Design review of the part built by this model. Coordinates are the model's own, in mm. A direction names the side the tool comes from. Give positions to 0.01 mm unless a question says otherwise; leave off trailing zeros. Write each loop counter-clockwise with the first axis right and the second up, starting at its lowest first coordinate (ties: lowest second). Pieces come first, ordered by that corner, then holes. Notation, with made-up numbers: (-33, -10.5) -> (-2, -10.5) arc R28 ccw to (-2, 21.5) -> close; hole circle Ø5 at (44, 3). An arc over 180 degrees is marked (long way). Answer as a JSON object with one key per item and string values.
```python
from build123d import *

# Parameters (mm, degrees)
SKETCH_1_W               = 150
SKETCH_1_H               = 60
EXTRUDE_1_DEPTH          = 30
CUT_EXTRUDE_1_DEPTH      = 100
CUT_EXTRUDE_2_DEPTH      = 165.316767252
CUT_EXTRUDE_2_DEPTH_BACK = 165.316767252
SKETCH_5_R               = 2.05


with BuildPart() as part:
    # 스케치1 → 보스-돌출1 (new, symmetric)
    with BuildSketch(Plane(origin=(0, 0, 0), x_dir=(0, 0, -1), z_dir=(1, 0, 0))):
        with Locations((75, -30)):
            Rectangle(SKETCH_1_W, SKETCH_1_H)
    extrude(amount=EXTRUDE_1_DEPTH, both=True)

    # 스케치4 → 컷-돌출1 (cut)
    with BuildSketch(Plane.XY):
        with BuildLine():
            Line((-22.575, -30), (-22.575, -60))
            Line((-22.575, -60), (22.575, -60))
            Line((22.575, -60), (22.575, -30))
            ThreePointArc((22.575, -30), (0, -7.425), (-22.575, -30))
        make_face()
    extrude(amount=-CUT_EXTRUDE_1_DEPTH, mode=Mode.SUBTRACT)

    # 스케치5 → 컷-돌출2 (cut, two sides: drawn at the far end of the back side and taken through both)
    with BuildSketch(Plane(origin=(0, 0, 0), x_dir=(0, 0, -1), z_dir=(1, 0, 0)).offset(-CUT_EXTRUDE_2_DEPTH_BACK)):
        with Locations((107.446436282, -43.174787846)):
            Circle(SKETCH_5_R)
        with Locations((139.331395941, -33.939123257)):
            Circle(SKETCH_5_R)
    extrude(amount=CUT_EXTRUDE_2_DEPTH + CUT_EXTRUDE_2_DEPTH_BACK, mode=Mode.SUBTRACT)


solid = part.part
```
(1) We need section A-A, the plane x = 0. State the section outline as (y, z) points (3 decimals), then the cut area to 3 significant figures.
Here are the results:
{"outline": "(-60, -150) -> (0, -150) -> (0, 0) -> (-7.425, 0) -> (-7.425, -100) -> (-60, -100) -> close; hole circle Ø4.1 at (-43.175, -107.446); hole circle Ø4.1 at (-33.939, -139.331)", "area": "3,720 mm²"}
(2) We need section C-C, the plane y = -55. State the section outline as (x, z) points (3 decimals), then the cut area to 4 significant figures.
Here are the results:
{"outline": "(-30, -150) -> (30, -150) -> (30, 0) -> (22.575, 0) -> (22.575, -100) -> (-22.575, -100) -> (-22.575, 0) -> (-30, 0) -> close", "area": "4,485 mm²"}
(3) For line 1 along Z through (x, y) = (-18, -43.5); line 2 along X through (y, z) = (-54.5, -67) (3 decimals); line 3 along Z through (x, y) = (-18, -34), list the stretches that pass through material, from the lowest coordinate up.
Here are the results:
{"line 1": "z = -150 to -109.47, -105.42 to -100", "line 2": "x = -30 to -22.575, 22.575 to 30", "line 3": "z = -150 to -141.38, -137.28 to -100"}
(4) The part is to be moulded in two halves that separate along Y. For faces 3 (the flat face through (30, -30, -74)), 4 (the cylindrical face through (-0.42, -41.446, -108.549)), 5 (the flat face through (0, -60, -107)), say which applies: +Y half, -Y half, draft (parallel to the pull), parting line (faces both ways), or undercut.
Here are the results:
{"face 3": "draft", "face 4": "undercut", "face 5": "-Y half"}
(5) We need section D-D, the plane z = -107.5. State the section outline as (x, y) points.
Here are the results:
{"outline": "(-30, -60) -> (30, -60) -> (30, -45.22) -> (-30, -45.22) -> close; (-30, -41.13) -> (30, -41.13) -> (30, 0) -> (-30, 0) -> close"}
(6) We need section B-B, the plane z = -24. State the section outline as (x, y) points (3 decimals).
Here are the results:
{"outline": "(-30, -60) -> (-22.575, -60) -> (-22.575, -30) arc R22.575 cw to (22.575, -30) -> (22.575, -60) -> (30, -60) -> (30, 0) -> (-30, 0) -> close"}
(7) For faces 1 (the flat face through (22.575, -45, -49)), 2 (the flat face through (0, 0, -74)), list the 3-axis set-ups (+Z, -Z, +X, -X, +Y, -Y) from which the entire face can be reached by the end or side of a thin tool; tool diameter is ignored.
Here are the results:
{"face 1": "+Z, -Y", "face 2": "+Z, -Z, +X, -X, +Y"}
(8) Clearance check with flat-ended pins moving along their axes: pin 1 (1.5 mm diameter, centred on x = -5.5, y = -23, fed in from +Z); pin 2 (1 mm diameter, centred on x = -8, z = -66.5, fed in from -Y); pin 3 (2.5 mm diameter, centred on y = -43.17, z = -107.45, fed in from -X). State where each tip first meets the part, or that it passes through.
Here are the results:
{"pin 1": "stops at z = -100", "pin 2": "stops at y = -9.09", "pin 3": "passes through"}
